Can you work these out from the model? Positions are in its coordinate system, mm. Coordinates: 2 decimals unless noted, no trailing zeros. Order: outer loops, then holes, each group sorted by start corner. A loop starts at its lowest first (then second) coordinate and runs counter-clockwise, first axis right, second up. Notation, with made-up numbers: M 76.5,34 L 83.5,34 A25 cw 83.5,70 Z; hole C -7.75,-17.5 d4. An arc over 180 degrees is marked long. Answer as a JSON object with one key per item and string values.
Autodesk Inventor part; units mm, degrees
ref_plane "YZ Plane" through (0, 0, 0) normal (1, 0, 0) x (0, 1, 0)
ref_plane "XZ Plane" through (0, 0, 0) normal (0, 1, 0) x (-1, 0, 0)
ref_plane "XY Plane" through (0, 0, 0) normal (0, 0, 1) x (1, 0, 0)
sketch "스케치1" plane through (0, 0, 0) normal (0, 0, 1) x (1, 0, 0)
  line L0 (90, -7) -> (-116, -7)
  line L1 (-116, -7) -> (-116, -57)
  line L2 (-116, -57) -> (90, -57)
  line L3 (90, -57) -> (90, -7)
  point P0 (0, 0)
  dimension "d0" = 50
  dimension "d3" = 206
extrude "돌출1" add sketch "스케치1" along normal blind 2
sketch "스케치2" plane through (0, 0, 2) normal (0, 0, 1) x (1, 0, 0)
  line L0 (90, -7) -> (-116, -7)
  line L1 (-115, -7) -> (-109.6, -7)
  line L2 (-109.6, -7) -> (-109.6, -57.0095)
  line L3 (-109.6, -57.0095) -> (-115, -57.0095)
  line L4 (-115, -57.0095) -> (-115, -7)
  line L5 (-116, -7) -> (-116, -57)
  line L6 (-116, -57) -> (90, -57)
  line L7 (83.6, -7) -> (89, -7)
  line L8 (89, -7) -> (89, -57)
  line L9 (89, -57) -> (83.6, -57)
  line L10 (83.6, -57) -> (83.6, -7)
  line L11 (90, -57) -> (90, -7)
  point P0 (0, 0)
  dimension "d4" = 5.4
  dimension "d5" = 1
  dimension "d6" = 5.4
  dimension "d7" = 1
extrude "돌출2" cut sketch "스케치2" against normal blind 1 contours L8 L6 L10 L0 | L2 L6 L4 L0 | L2 L3 L4 L6
sketch "스케치3" plane through (0, 0, 2) normal (0, 0, 1) x (1, 0, 0)
  line L0 (83.6, -57) -> (83.6, -7)
  line L1 (83.6, -7) -> (-109.6, -7)
  line L2 (-109.6, -7) -> (-109.6, -57)
  line L3 (-109.6, -57) -> (83.6, -57)
  line L4 (-109.6, -29.3333) -> (-64.6, -29.3333)
  line L5 (83.6, -24) -> (38.6, -24)
  line L6 (90, -7) -> (-116, -7)
  line L7 (-13, -7) -> (-13, -12)
  line L8 (-13, -12) -> (-63.6, -12)
  line L9 (-109.6, -7) -> (-109.6, -57)
  line L10 (9.6, -12) -> (37.6, -12)
  line L11 (38.6, -26) -> (38.6, -13)
  line L12 (-64.6, -26) -> (-64.6, -13)
  line L13 (37.6, -12) -> (9.6, -12)
  line L14 (8.6, -13) -> (8.6, -26)
  line L15 (9.6, -27) -> (37.6, -27)
  line L16 (38.6, -26) -> (38.6, -13)
  line L17 (-63.6, -12) -> (-35.6, -12)
  line L18 (-34.6, -13) -> (-34.6, -26)
  line L19 (-35.6, -27) -> (-63.6, -27)
  line L20 (-64.6, -26) -> (-64.6, -13)
  arc A0 (-34.6, -13) -> (-35.6, -12) centre (-35.6, -13) ccw
  arc A1 (-35.6, -27) -> (-34.6, -26) centre (-35.6, -26) ccw
  arc A2 (-64.6, -26) -> (-63.6, -27) centre (-63.6, -26) ccw
  arc A3 (-63.6, -12) -> (-64.6, -13) centre (-63.6, -13) ccw
  arc A4 (9.6, -12) -> (8.6, -13) centre (9.6, -13) ccw
  arc A5 (38.6, -13) -> (37.6, -12) centre (37.6, -13) ccw
  arc A6 (37.6, -27) -> (38.6, -26) centre (37.6, -26) ccw
  arc A7 (8.6, -26) -> (9.6, -27) centre (9.6, -26) ccw
  point P0 (0, 0)
  point P1 (83.6, -12)
  point P2 (38.6, -12)
  point P3 (-64.6, -12)
  point P4 (8.6, -27)
  point P5 (8.6, -12)
  point P6 (38.6, -27)
  point P7 (-34.6, -27)
  point P8 (-34.6, -12)
  point P9 (-64.6, -27)
  dimension "d10" = 45
  dimension "d11" = 45
  dimension "d12" = 5
  dimension "d13" = 30
  dimension "d14" = 15
  dimension "d15" = 30
  dimension "d16" = 15
  dimension "d19" = 1
extrude "돌출3" cut sketch "스케치3" against normal blind 10 contours L11 A6 L15 A7 L14 A4 L10 A5 | A0 L18 A1 L19 A2 L12 A3 L8
properties part number "뒷판" material "알루미늄 6061"
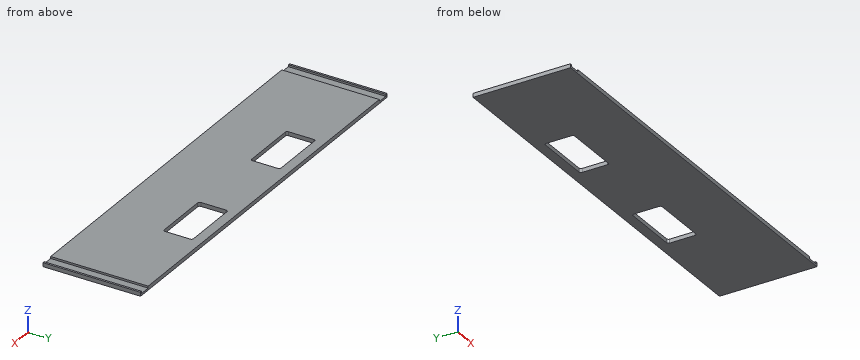
Item 1: I'm going to push a flat-ended pin straight in: pin 1 (2.5 mm diameter, centred on x = -111, y = -43, fed in from +Z). Where does the tip first touch, or does it pass through?
Answers follow:
{"pin 1": "stops at z = 1"}
Item 2: I want a section at B-B, the plane x = -53.5. Write out the boundary of the cut face in (y, z).
Answers follow:
{"outline": "M -57,0 L -27,0 L -27,2 L -57,2 Z; M -12,0 L -7,0 L -7,2 L -12,2 Z"}
Item 3: I want a section at C-C, the plane y = -17. Write out the boundary of the cut face in (x, z).
Answers follow:
{"outline": "M -116,0 L -64.6,0 L -64.6,2 L -109.6,2 L -109.6,1 L -115,1 L -115,2 L -116,2 Z; M -34.6,0 L 8.6,0 L 8.6,2 L -34.6,2 Z; M 38.6,0 L 90,0 L 90,2 L 89,2 L 89,1 L 83.6,1 L 83.6,2 L 38.6,2 Z"}
Item 4: I want a section at D-D, the plane y = -50.5. Write out the boundary of the cut face in (x, z), plus the area to 3 significant figures.
Answers follow:
{"outline": "M -116,0 L 90,0 L 90,2 L 89,2 L 89,1 L 83.6,1 L 83.6,2 L -109.6,2 L -109.6,1 L -115,1 L -115,2 L -116,2 Z", "area": "401 mm^2"}
Item 5: I want a section at A-A, the plane z = 1.5. Write out the boundary of the cut face in (x, y), plus the area to 3 significant figures.
Answers follow:
{"outline": "M -116,-57 L -115,-57 L -115,-7 L -116,-7 Z; M -109.6,-57 L 83.6,-57 L 83.6,-7 L -109.6,-7 Z; M 89,-57 L 90,-57 L 90,-7 L 89,-7 Z; hole M -64.6,-26 A1 ccw -63.6,-27 L -35.6,-27 A1 ccw -34.6,-26 L -34.6,-13 A1 ccw -35.6,-12 L -63.6,-12 A1 ccw -64.6,-13 Z; hole M 8.6,-26 A1 ccw 9.6,-27 L 37.6,-27 A1 ccw 38.6,-26 L 38.6,-13 A1 ccw 37.6,-12 L 9.6,-12 A1 ccw 8.6,-13 Z", "area": "8,860 mm^2"}
Item 6: Please list where these lines run through material, in increasing order: line 1 (X direction, y = -49, z = 1.25); line 2 (X direction, y = -20.5, z = 0.2); line 3 (X direction, y = -23, z = 1.1).
Answers follow:
{"line 1": "x = -116 to -115, -109.6 to 83.6, 89 to 90", "line 2": "x = -116 to -64.6, -34.6 to 8.6, 38.6 to 90", "line 3": "x = -116 to -115, -109.6 to -64.6, -34.6 to 8.6, 38.6 to 83.6, 89 to 90"}
